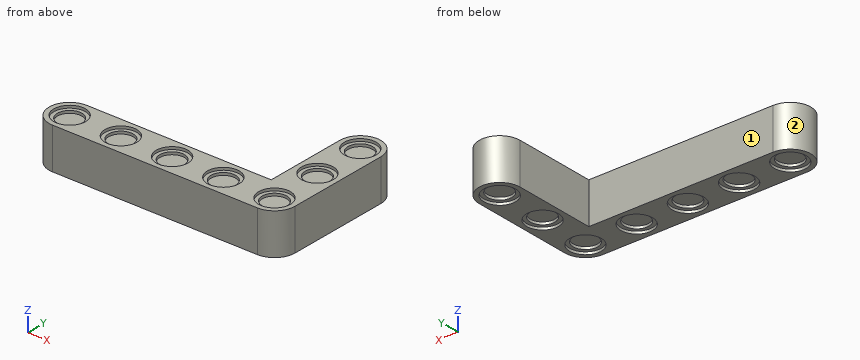
from build123d import *

# Parameters (mm, degrees)
BOSS_EXTRUDE1_DEPTH      = 8
SKETCH2_R                = 2.4
CUT_EXTRUDE1_DEPTH       = 1
SKETCH3_R                = 3.1
CUT_EXTRUDE2_DEPTH       = 0.5
LPATTERN1_COUNT          = 5
LPATTERN1_PITCH          = 10
LPATTERN1_COUNT_DIR2     = 3
LPATTERN1_PITCH_DIR2     = 10
MIRROR1_COPY_1_SKETCH_R  = 2.4
MIRROR1_COPY_1_DEPTH     = 1
MIRROR1_COPY_2_SKETCH_R  = 2.4
MIRROR1_COPY_2_DEPTH     = 1
MIRROR1_COPY_3_SKETCH_R  = 2.4
MIRROR1_COPY_3_DEPTH     = 1
MIRROR1_COPY_4_SKETCH_R  = 2.4
MIRROR1_COPY_4_DEPTH     = 1
MIRROR1_COPY_5_SKETCH_R  = 2.4
MIRROR1_COPY_5_DEPTH     = 1
MIRROR1_COPY_6_SKETCH_R  = 2.4
MIRROR1_COPY_6_DEPTH     = 1
MIRROR1_COPY_7_SKETCH_R  = 2.4
MIRROR1_COPY_7_DEPTH     = 1
MIRROR1_COPY_8_SKETCH_R  = 2.4
MIRROR1_COPY_8_DEPTH     = 1
MIRROR1_COPY_9_SKETCH_R  = 2.4
MIRROR1_COPY_9_DEPTH     = 1
MIRROR1_COPY_10_SKETCH_R = 2.4
MIRROR1_COPY_10_DEPTH    = 1
MIRROR1_COPY_11_SKETCH_R = 2.4
MIRROR1_COPY_11_DEPTH    = 1
MIRROR1_COPY_12_SKETCH_R = 2.4
MIRROR1_COPY_12_DEPTH    = 1
MIRROR1_COPY_13_SKETCH_R = 2.4
MIRROR1_COPY_13_DEPTH    = 1
MIRROR1_COPY_14_SKETCH_R = 2.4
MIRROR1_COPY_14_DEPTH    = 1
MIRROR1_COPY_15_SKETCH_R = 3.1
MIRROR1_COPY_15_DEPTH    = 0.5
MIRROR1_COPY_16_SKETCH_R = 3.1
MIRROR1_COPY_16_DEPTH    = 0.5
MIRROR1_COPY_17_SKETCH_R = 3.1
MIRROR1_COPY_17_DEPTH    = 0.5
MIRROR1_COPY_18_SKETCH_R = 3.1
MIRROR1_COPY_18_DEPTH    = 0.5
MIRROR1_COPY_19_SKETCH_R = 3.1
MIRROR1_COPY_19_DEPTH    = 0.5
MIRROR1_COPY_20_SKETCH_R = 3.1
MIRROR1_COPY_20_DEPTH    = 0.5
MIRROR1_COPY_21_SKETCH_R = 3.1
MIRROR1_COPY_21_DEPTH    = 0.5
MIRROR1_COPY_22_SKETCH_R = 3.1
MIRROR1_COPY_22_DEPTH    = 0.5
MIRROR1_COPY_23_SKETCH_R = 3.1
MIRROR1_COPY_23_DEPTH    = 0.5
MIRROR1_COPY_24_SKETCH_R = 3.1
MIRROR1_COPY_24_DEPTH    = 0.5
MIRROR1_COPY_25_SKETCH_R = 3.1
MIRROR1_COPY_25_DEPTH    = 0.5
MIRROR1_COPY_26_SKETCH_R = 3.1
MIRROR1_COPY_26_DEPTH    = 0.5
MIRROR1_COPY_27_SKETCH_R = 3.1
MIRROR1_COPY_27_DEPTH    = 0.5
MIRROR1_COPY_28_SKETCH_R = 3.1
MIRROR1_COPY_28_DEPTH    = 0.5


with BuildPart() as part:
    # Sketch1 → Boss-Extrude1 (new body)
    with BuildSketch(Plane.XY):
        with BuildLine():
            Line((0, 4), (36, 4))
            Line((36, 4), (36, 20))
            ThreePointArc((36, 20), (40, 24), (44, 20))
            Line((44, 20), (44, 0))
            ThreePointArc((44, 0), (42.828427125, -2.828427125), (40, -4))
            Line((40, -4), (0, -4))
            ThreePointArc((0, -4), (-4, 0), (0, 4))
        make_face()
    extrude(amount=-BOSS_EXTRUDE1_DEPTH)

    # Sketch2 → Cut-Extrude1 (cut)
    with BuildSketch(Plane.XY):
        Circle(SKETCH2_R)
    cut_extrude1 = extrude(amount=-CUT_EXTRUDE1_DEPTH, mode=Mode.SUBTRACT)

    # Sketch3 → Cut-Extrude2 (cut)
    with BuildSketch(Plane.XY):
        Circle(SKETCH3_R)
    cut_extrude2 = extrude(amount=-CUT_EXTRUDE2_DEPTH, mode=Mode.SUBTRACT)

    # LPattern1: Cut-Extrude1, Cut-Extrude2 5 × 3
    with Locations(*[(i * LPATTERN1_PITCH, j * LPATTERN1_PITCH_DIR2, 0) for i in range(LPATTERN1_COUNT) for j in range(LPATTERN1_COUNT_DIR2) if (i, j) != (0, 0)]):
        add(cut_extrude1, mode=Mode.SUBTRACT)
        add(cut_extrude2, mode=Mode.SUBTRACT)

    # Mirror1: Cut-Extrude1, Cut-Extrude2 across plane
    add(cut_extrude1.mirror(Plane.XY.offset(-4)), mode=Mode.SUBTRACT)
    add(cut_extrude2.mirror(Plane.XY.offset(-4)), mode=Mode.SUBTRACT)

    # Mirror1 copy 1 sketch → Mirror1 copy 1 (cut)
    with BuildSketch(Plane(origin=(0, 10, -8), x_dir=(1, 0, 0), z_dir=(0, 0, -1))):
        Circle(MIRROR1_COPY_1_SKETCH_R)
    extrude(amount=-MIRROR1_COPY_1_DEPTH, mode=Mode.SUBTRACT)

    # Mirror1 copy 2 sketch → Mirror1 copy 2 (cut)
    with BuildSketch(Plane(origin=(0, 20, -8), x_dir=(1, 0, 0), z_dir=(0, 0, -1))):
        Circle(MIRROR1_COPY_2_SKETCH_R)
    extrude(amount=-MIRROR1_COPY_2_DEPTH, mode=Mode.SUBTRACT)

    # Mirror1 copy 3 sketch → Mirror1 copy 3 (cut)
    with BuildSketch(Plane(origin=(10, 0, -8), x_dir=(1, 0, 0), z_dir=(0, 0, -1))):
        Circle(MIRROR1_COPY_3_SKETCH_R)
    extrude(amount=-MIRROR1_COPY_3_DEPTH, mode=Mode.SUBTRACT)

    # Mirror1 copy 4 sketch → Mirror1 copy 4 (cut)
    with BuildSketch(Plane(origin=(10, 10, -8), x_dir=(1, 0, 0), z_dir=(0, 0, -1))):
        Circle(MIRROR1_COPY_4_SKETCH_R)
    extrude(amount=-MIRROR1_COPY_4_DEPTH, mode=Mode.SUBTRACT)

    # Mirror1 copy 5 sketch → Mirror1 copy 5 (cut)
    with BuildSketch(Plane(origin=(10, 20, -8), x_dir=(1, 0, 0), z_dir=(0, 0, -1))):
        Circle(MIRROR1_COPY_5_SKETCH_R)
    extrude(amount=-MIRROR1_COPY_5_DEPTH, mode=Mode.SUBTRACT)

    # Mirror1 copy 6 sketch → Mirror1 copy 6 (cut)
    with BuildSketch(Plane(origin=(20, 0, -8), x_dir=(1, 0, 0), z_dir=(0, 0, -1))):
        Circle(MIRROR1_COPY_6_SKETCH_R)
    extrude(amount=-MIRROR1_COPY_6_DEPTH, mode=Mode.SUBTRACT)

    # Mirror1 copy 7 sketch → Mirror1 copy 7 (cut)
    with BuildSketch(Plane(origin=(20, 10, -8), x_dir=(1, 0, 0), z_dir=(0, 0, -1))):
        Circle(MIRROR1_COPY_7_SKETCH_R)
    extrude(amount=-MIRROR1_COPY_7_DEPTH, mode=Mode.SUBTRACT)

    # Mirror1 copy 8 sketch → Mirror1 copy 8 (cut)
    with BuildSketch(Plane(origin=(20, 20, -8), x_dir=(1, 0, 0), z_dir=(0, 0, -1))):
        Circle(MIRROR1_COPY_8_SKETCH_R)
    extrude(amount=-MIRROR1_COPY_8_DEPTH, mode=Mode.SUBTRACT)

    # Mirror1 copy 9 sketch → Mirror1 copy 9 (cut)
    with BuildSketch(Plane(origin=(30, 0, -8), x_dir=(1, 0, 0), z_dir=(0, 0, -1))):
        Circle(MIRROR1_COPY_9_SKETCH_R)
    extrude(amount=-MIRROR1_COPY_9_DEPTH, mode=Mode.SUBTRACT)

    # Mirror1 copy 10 sketch → Mirror1 copy 10 (cut)
    with BuildSketch(Plane(origin=(30, 10, -8), x_dir=(1, 0, 0), z_dir=(0, 0, -1))):
        Circle(MIRROR1_COPY_10_SKETCH_R)
    extrude(amount=-MIRROR1_COPY_10_DEPTH, mode=Mode.SUBTRACT)

    # Mirror1 copy 11 sketch → Mirror1 copy 11 (cut)
    with BuildSketch(Plane(origin=(30, 20, -8), x_dir=(1, 0, 0), z_dir=(0, 0, -1))):
        Circle(MIRROR1_COPY_11_SKETCH_R)
    extrude(amount=-MIRROR1_COPY_11_DEPTH, mode=Mode.SUBTRACT)

    # Mirror1 copy 12 sketch → Mirror1 copy 12 (cut)
    with BuildSketch(Plane(origin=(40, 0, -8), x_dir=(1, 0, 0), z_dir=(0, 0, -1))):
        Circle(MIRROR1_COPY_12_SKETCH_R)
    extrude(amount=-MIRROR1_COPY_12_DEPTH, mode=Mode.SUBTRACT)

    # Mirror1 copy 13 sketch → Mirror1 copy 13 (cut)
    with BuildSketch(Plane(origin=(40, 10, -8), x_dir=(1, 0, 0), z_dir=(0, 0, -1))):
        Circle(MIRROR1_COPY_13_SKETCH_R)
    extrude(amount=-MIRROR1_COPY_13_DEPTH, mode=Mode.SUBTRACT)

    # Mirror1 copy 14 sketch → Mirror1 copy 14 (cut)
    with BuildSketch(Plane(origin=(40, 20, -8), x_dir=(1, 0, 0), z_dir=(0, 0, -1))):
        Circle(MIRROR1_COPY_14_SKETCH_R)
    extrude(amount=-MIRROR1_COPY_14_DEPTH, mode=Mode.SUBTRACT)

    # Mirror1 copy 15 sketch → Mirror1 copy 15 (cut)
    with BuildSketch(Plane(origin=(0, 10, -8), x_dir=(1, 0, 0), z_dir=(0, 0, -1))):
        Circle(MIRROR1_COPY_15_SKETCH_R)
    extrude(amount=-MIRROR1_COPY_15_DEPTH, mode=Mode.SUBTRACT)

    # Mirror1 copy 16 sketch → Mirror1 copy 16 (cut)
    with BuildSketch(Plane(origin=(0, 20, -8), x_dir=(1, 0, 0), z_dir=(0, 0, -1))):
        Circle(MIRROR1_COPY_16_SKETCH_R)
    extrude(amount=-MIRROR1_COPY_16_DEPTH, mode=Mode.SUBTRACT)

    # Mirror1 copy 17 sketch → Mirror1 copy 17 (cut)
    with BuildSketch(Plane(origin=(10, 0, -8), x_dir=(1, 0, 0), z_dir=(0, 0, -1))):
        Circle(MIRROR1_COPY_17_SKETCH_R)
    extrude(amount=-MIRROR1_COPY_17_DEPTH, mode=Mode.SUBTRACT)

    # Mirror1 copy 18 sketch → Mirror1 copy 18 (cut)
    with BuildSketch(Plane(origin=(10, 10, -8), x_dir=(1, 0, 0), z_dir=(0, 0, -1))):
        Circle(MIRROR1_COPY_18_SKETCH_R)
    extrude(amount=-MIRROR1_COPY_18_DEPTH, mode=Mode.SUBTRACT)

    # Mirror1 copy 19 sketch → Mirror1 copy 19 (cut)
    with BuildSketch(Plane(origin=(10, 20, -8), x_dir=(1, 0, 0), z_dir=(0, 0, -1))):
        Circle(MIRROR1_COPY_19_SKETCH_R)
    extrude(amount=-MIRROR1_COPY_19_DEPTH, mode=Mode.SUBTRACT)

    # Mirror1 copy 20 sketch → Mirror1 copy 20 (cut)
    with BuildSketch(Plane(origin=(20, 0, -8), x_dir=(1, 0, 0), z_dir=(0, 0, -1))):
        Circle(MIRROR1_COPY_20_SKETCH_R)
    extrude(amount=-MIRROR1_COPY_20_DEPTH, mode=Mode.SUBTRACT)

    # Mirror1 copy 21 sketch → Mirror1 copy 21 (cut)
    with BuildSketch(Plane(origin=(20, 10, -8), x_dir=(1, 0, 0), z_dir=(0, 0, -1))):
        Circle(MIRROR1_COPY_21_SKETCH_R)
    extrude(amount=-MIRROR1_COPY_21_DEPTH, mode=Mode.SUBTRACT)

    # Mirror1 copy 22 sketch → Mirror1 copy 22 (cut)
    with BuildSketch(Plane(origin=(20, 20, -8), x_dir=(1, 0, 0), z_dir=(0, 0, -1))):
        Circle(MIRROR1_COPY_22_SKETCH_R)
    extrude(amount=-MIRROR1_COPY_22_DEPTH, mode=Mode.SUBTRACT)

    # Mirror1 copy 23 sketch → Mirror1 copy 23 (cut)
    with BuildSketch(Plane(origin=(30, 0, -8), x_dir=(1, 0, 0), z_dir=(0, 0, -1))):
        Circle(MIRROR1_COPY_23_SKETCH_R)
    extrude(amount=-MIRROR1_COPY_23_DEPTH, mode=Mode.SUBTRACT)

    # Mirror1 copy 24 sketch → Mirror1 copy 24 (cut)
    with BuildSketch(Plane(origin=(30, 10, -8), x_dir=(1, 0, 0), z_dir=(0, 0, -1))):
        Circle(MIRROR1_COPY_24_SKETCH_R)
    extrude(amount=-MIRROR1_COPY_24_DEPTH, mode=Mode.SUBTRACT)

    # Mirror1 copy 25 sketch → Mirror1 copy 25 (cut)
    with BuildSketch(Plane(origin=(30, 20, -8), x_dir=(1, 0, 0), z_dir=(0, 0, -1))):
        Circle(MIRROR1_COPY_25_SKETCH_R)
    extrude(amount=-MIRROR1_COPY_25_DEPTH, mode=Mode.SUBTRACT)

    # Mirror1 copy 26 sketch → Mirror1 copy 26 (cut)
    with BuildSketch(Plane(origin=(40, 0, -8), x_dir=(1, 0, 0), z_dir=(0, 0, -1))):
        Circle(MIRROR1_COPY_26_SKETCH_R)
    extrude(amount=-MIRROR1_COPY_26_DEPTH, mode=Mode.SUBTRACT)

    # Mirror1 copy 27 sketch → Mirror1 copy 27 (cut)
    with BuildSketch(Plane(origin=(40, 10, -8), x_dir=(1, 0, 0), z_dir=(0, 0, -1))):
        Circle(MIRROR1_COPY_27_SKETCH_R)
    extrude(amount=-MIRROR1_COPY_27_DEPTH, mode=Mode.SUBTRACT)

    # Mirror1 copy 28 sketch → Mirror1 copy 28 (cut)
    with BuildSketch(Plane(origin=(40, 20, -8), x_dir=(1, 0, 0), z_dir=(0, 0, -1))):
        Circle(MIRROR1_COPY_28_SKETCH_R)
    extrude(amount=-MIRROR1_COPY_28_DEPTH, mode=Mode.SUBTRACT)


solid = part.part
The listing builds one solid part. Answer for the finished solid, in the listing's coordinates (mm). Face numbers are marked on the shaded views. A direction names the side the tool comes from. Round coordinates to 2 decimals unless told otherwise and drop trailing zeros. Loops run counter-clockwise (first coordinate to the right, second up) from the corner with the lowest first, then second, coordinate; pieces in that order, holes last. Notation, with made-up numbers: M 2,47.25 L 51,47.25 A18 cw 51,73.25 Z; hole C 63,-36.75 d2. An arc over 180 degrees is marked long. Write each question's results on one line, items separated by ' | '. Start each with the question number.
1) Find section A-A on y = 10. Write down the section's boundary in (x, z), plus the area to 3 significant figures.
2) Each of these flat-tipped pins is pushed along its axis until it touches: pin 1 (1.9 mm diameter, centred on x = 11, y = 0.5, fed in from +Z); pin 2 (4 mm diameter, centred on y = 4, z = -3, fed in from -X); pin 3 (6 mm diameter, centred on x = 10, y = 0, fed in from -Z). Where does it stop, or does it pass through?
3) Which of the six approach directions +Z, -Z, +X, -X, +Y, -Y give full straight-line access (tool end or side, diameter ignored) to the marked faces 1 and 2?
4) Find section B-B on x = 30. Write down the section's boundary in (y, z), plus the area to 3 significant figures.
5) Straight lines are drawn through the part: probe 1 along X at (y, z) = (0, -7.2); probe 2 along Y at (x, z) = (40, -7.55); probe 3 along Y at (x, z) = (0, -0.75). For each, find the intervals that lie inside material, in ascending order.
6) Find section D-D on x = 24. Write down the section's boundary in (y, z).
7) Find section C-C on z = -1.5. Write down the section's boundary in (x, y), plus the area to 3 significant figures.
Final values:
1) outline: M 36,-8 L 36.9,-8 L 36.9,-7.5 L 37.6,-7.5 L 37.6,-7 L 42.4,-7 L 42.4,-7.5 L 43.1,-7.5 L 43.1,-8 L 44,-8 L 44,0 L 43.1,0 L 43.1,-0.5 L 42.4,-0.5 L 42.4,-1 L 37.6,-1 L 37.6,-0.5 L 36.9,-0.5 L 36.9,0 L 36,0 Z | area: 53.0 mm²
2) pin 1: z = -1 | pin 2: x = -3.46 | pin 3: z = -7.5
3) face 1: +Z, -Z, -X, +Y | face 2: +Z, -Z, -X
4) outline: M -4,-8 L -3.1,-8 L -3.1,-7.5 L -2.4,-7.5 L -2.4,-7 L 2.4,-7 L 2.4,-7.5 L 3.1,-7.5 L 3.1,-8 L 4,-8 L 4,0 L 3.1,0 L 3.1,-0.5 L 2.4,-0.5 L 2.4,-1 L -2.4,-1 L -2.4,-0.5 L -3.1,-0.5 L -3.1,0 L -4,0 Z | area: 53.0 mm²
5) probe 1: -4 to -2.4, 2.4 to 7.6, 12.4 to 17.6, 22.4 to 27.6, 32.4 to 37.6, 42.4 to 44 | probe 2: -4 to -3.1, 3.1 to 6.9, 13.1 to 16.9, 23.1 to 24 | probe 3: -4 to -2.4, 2.4 to 4
6) outline: M -4,-8 L 4,-8 L 4,0 L -4,0 Z
7) outline: M 0,-4 L 40,-4 A4 ccw 44,0 L 44,20 A4 ccw 36,20 L 36,4 L 0,4 A4 ccw Z | area: 527 mm²
